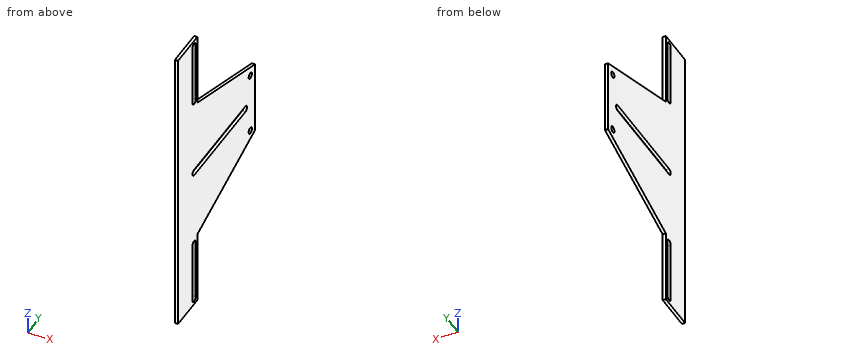
```python
from build123d import *

# Parameters (mm, degrees)
SKETCH1_R           = 6.35
BOSS_EXTRUDE1_DEPTH = 6.35


with BuildPart() as part:
    # Sketch1 → Boss-Extrude1 (new body)
    with BuildSketch(Plane(origin=(0, 0, 0), x_dir=(0, 0, -1), z_dir=(1, 0, 0))):
        Polygon((304.8, 0), (-304.8, 0), (-304.8, 76.2), (-152.4, 76.2), (-76.2, 304.8), (76.2, 304.8), (152.4, 76.2), (304.8, 76.2), align=None)
        with Locations((-63.5, 285.75)):
            Circle(SKETCH1_R, mode=Mode.SUBTRACT)
        with Locations(Location((63.5, 285.75, 0), (0, 0, 180))):
            Circle(SKETCH1_R, mode=Mode.SUBTRACT)
        with BuildLine():
            Line((-292.1, 69.85), (-165.1, 69.85))
            ThreePointArc((-165.1, 69.85), (-158.75, 63.5), (-165.1, 57.15))
            Line((-165.1, 57.15), (-292.1, 57.15))
            ThreePointArc((-292.1, 57.15), (-298.45, 63.5), (-292.1, 69.85))
        make_face(mode=Mode.SUBTRACT)
        with BuildLine():
            Line((292.1, 69.85), (165.1, 69.85))
            ThreePointArc((165.1, 69.85), (158.75, 63.5), (165.1, 57.15))
            Line((165.1, 57.15), (292.1, 57.15))
            ThreePointArc((292.1, 57.15), (298.45, 63.5), (292.1, 69.85))
        make_face(mode=Mode.SUBTRACT)
        with BuildLine():
            Line((6.35, 266.7), (6.35, 63.5))
            ThreePointArc((6.35, 63.5), (0, 57.15), (-6.35, 63.5))
            Line((-6.35, 63.5), (-6.35, 266.7))
            ThreePointArc((-6.35, 266.7), (0, 273.05), (6.35, 266.7))
        make_face(mode=Mode.SUBTRACT)
    extrude(amount=BOSS_EXTRUDE1_DEPTH)


solid = part.part
```
Model file for the job. Use its own axes, mm. Give positions to 0.01 mm unless a question says otherwise; leave off trailing zeros. Order: outer loops, then holes, each group sorted by start corner. A loop starts at its lowest first (then second) coordinate and runs counter-clockwise, first axis right, second up.
1) Saw through at C-C, the plane y = 131.5. Write the cut outline in (x, z).
2) Saw through at B-B, the plane z = 63.5. Write the cut outline in (x, y).
3) Pin check, flat tips, straight feed: pin 1 (1.5 mm diameter, centred on x = 5.5, y = 101, fed in from +Z); pin 2 (1.5 mm diameter, centred on x = 1, y = 171, fed in from +Z); pin 3 (1 mm diameter, centred on x = 4.5, y = 103.5, fed in from +Z). Stop position of each tip, or through.
4) Saw through at A-A, the plane x = 2.5. Write the cut outline in (y, z).
5) Wall check: probe 1 along Z at (x, y) = (4.5, 285.75); probe 2 along Y at (x, z) = (2.25, -63.5); probe 3 along Z at (x, y) = (5, 209). Give the ranges that are in metal, low to high.
Computed:
1. outline: (0, -133.97) - (6.35, -133.97) - (6.35, -6.35) - (0, -6.35) - close; (0, 6.35) - (6.35, 6.35) - (6.35, 133.97) - (0, 133.97) - close
2. outline: (0, 0) - (6.35, 0) - (6.35, 279.4) - (0, 279.4) - close; (0, 292.1) - (6.35, 292.1) - (6.35, 304.8) - (0, 304.8) - close
3. pin 1: stops at z = 144.38
3. pin 2: stops at z = 121.05
3. pin 3: stops at z = 143.47
4. outline: (0, -304.8) - (76.2, -304.8) - (76.2, -152.4) - (304.8, -76.2) - (304.8, 76.2) - (76.2, 152.4) - (76.2, 304.8) - (0, 304.8) - close; hole (57.15, -292.1) arc R6.35 ccw to (69.85, -292.1) - (69.85, -165.1) arc R6.35 ccw to (57.15, -165.1) - close; hole (57.15, 165.1) arc R6.35 ccw to (69.85, 165.1) - (69.85, 292.1) arc R6.35 ccw to (57.15, 292.1) - close; hole (63.5, -6.35) - (266.7, -6.35) arc R6.35 ccw to (266.7, 6.35) - (63.5, 6.35) arc R6.35 ccw to start; hole circle Ø12.7 at (285.75, -63.5); hole circle Ø12.7 at (285.75, 63.5)
5. probe 1: z = -82.55 to -69.85, -57.15 to 57.15, 69.85 to 82.55
5. probe 2: y = 0 to 279.4, 292.1 to 304.8
5. probe 3: z = -108.13 to -6.35, 6.35 to 108.13
